Verification items for this drawing (mm, ordinates from the low corner). Give positions to 0.01 mm unless a question says otherwise; leave off trailing zeros. Loops run counter-clockwise (first coordinate to the right, second up) from the corner with the lowest first, then second, coordinate; pieces in that order, holes last. Notation, with made-up numbers: (87, 11.25) -> (117, 11.25) arc R32 ccw to (117, 50.25) -> close; hole circle Ø9 at (40.25, 84.5). An arc over 180 degrees is marked (long way). Write each question's results on one line, items separated by ' | '. Start each with the question number.
Item 1: Scan lines: line 1 along Z through (x, y) = (152.5, 17.5); line 2 along Z through (x, y) = (194, 5); line 3 along Z through (x, y) = (168, 11). Record each from-to range of solid material in increasing order.
Item 2: Gauge pin test, flat ends, axial feed: pin 1 Ø5 at (y, z) = (11, 243.5) entering from -X; pin 2 Ø5.5 at (x, y) = (209.5, 11.5) entering from +Z; pin 3 Ø8 at (y, z) = (13, 359) entering from -X; pin 4 Ø2 at (x, z) = (142.5, 80.5) entering from -Y. Record the tip position at first contact, or that the pin passes through.
Item 3: Cross-section at C-C on z = 338. Enter the section's corners in (x, y).
Item 4: Cross-section at B-B on y = 8.25. Enter the section's corners in (x, z).
Item 5: Cross-section at D-D on x = 273. Enter the section's corners in (y, z).
Item 6: Cross-section at A-A on x = 203.5. Enter the section's corners in (y, z), then the cut area to 3 significant figures.
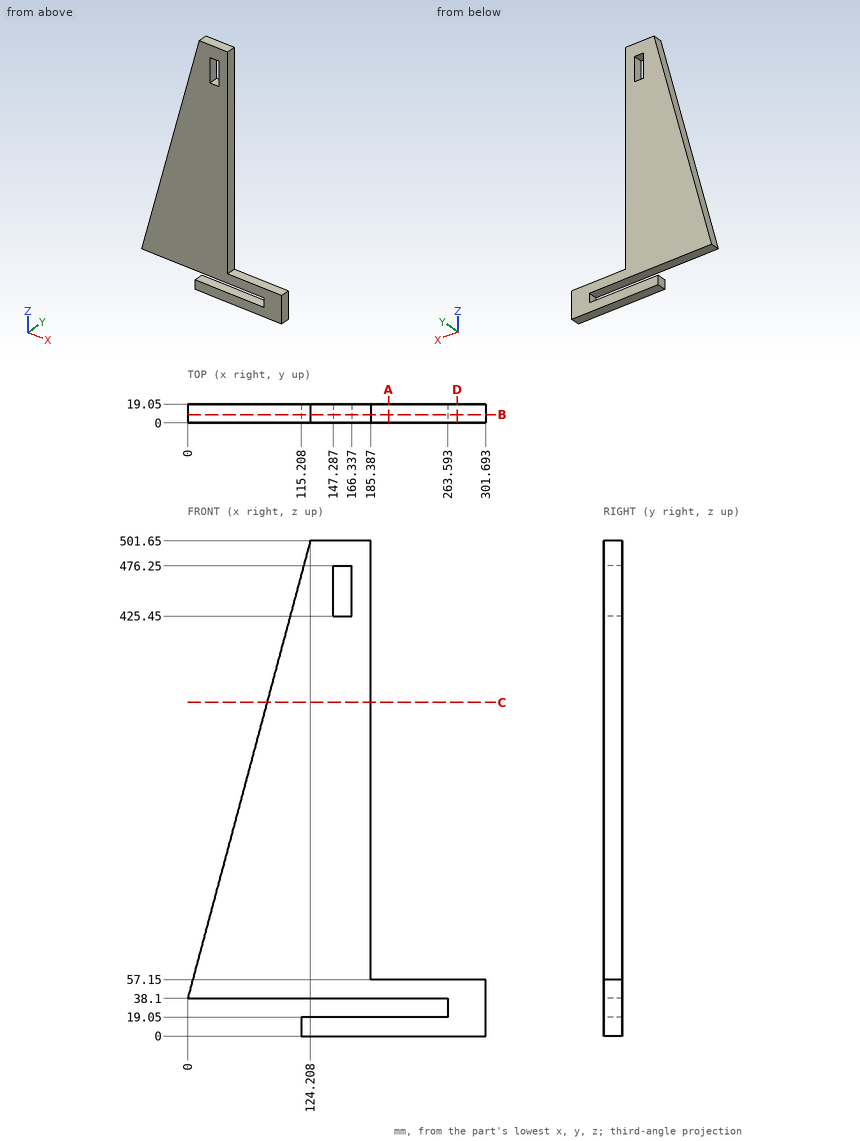
Answer sheet:
1) line 1: z = 0 to 19.05, 38.1 to 425.45, 476.25 to 501.65 | line 2: z = 0 to 19.05, 38.1 to 57.15 | line 3: z = 0 to 19.05, 38.1 to 501.65
2) pin 1: stops at x = 54.37 | pin 2: stops at z = 57.15 | pin 3: stops at x = 84.91 | pin 4: stops at y = 0
3) outline: (80.36, 0) -> (185.39, 0) -> (185.39, 19.05) -> (80.36, 19.05) -> close
4) outline: (0, 38.1) -> (263.59, 38.1) -> (263.59, 19.05) -> (115.21, 19.05) -> (115.21, 0) -> (301.69, 0) -> (301.69, 57.15) -> (185.39, 57.15) -> (185.39, 501.65) -> (124.21, 501.65) -> close; hole (147.29, 425.45) -> (166.34, 425.45) -> (166.34, 476.25) -> (147.29, 476.25) -> close
5) outline: (0, 0) -> (19.05, 0) -> (19.05, 57.15) -> (0, 57.15) -> close
6) outline: (0, 0) -> (19.05, 0) -> (19.05, 19.05) -> (0, 19.05) -> close; (0, 38.1) -> (19.05, 38.1) -> (19.05, 57.15) -> (0, 57.15) -> close | area: 726 mm²
